Design review of the part built by this model. Coordinates are the model's own, in mm. A direction names the side the tool comes from. Round coordinates to 2 decimals unless told otherwise and drop trailing zeros. Order: outer loops, then holes, each group sorted by start corner. A loop starts at its lowest first (then second) coordinate and runs counter-clockwise, first axis right, second up.
from build123d import *

# Parameters (mm, degrees)
F0_R           = 11
F0_R_2         = 2.5
F1_DEPTH       = 7
F2_D           = 5.5
F2_CSINK_D     = 11.2
F2_CSINK_ANGLE = 90
F4_DEPTH       = 36
F5_SIZE        = 32


with BuildPart() as f1:
    # F0 (on Front) → F1 (new body)
    with BuildSketch(Plane.XZ):
        with BuildLine():
            Line((0, -33), (127, -33))
            Line((127, -33), (127, 33))
            Line((127, 33), (-33, 33))
            Line((-33, 33), (-33, 0))
            ThreePointArc((-33, 0), (-23.3345237792, -23.3345237792), (0, -33))
        make_face()
        Circle(F0_R, mode=Mode.SUBTRACT)
        with Locations((67, 10)):
            Circle(F0_R_2, mode=Mode.SUBTRACT)
        with Locations((92, 10)):
            Circle(F0_R_2, mode=Mode.SUBTRACT)
        with Locations((117, 10)):
            Circle(F0_R_2, mode=Mode.SUBTRACT)
    extrude(amount=-F1_DEPTH)

    # F2 (through all)
    with Locations(Plane.XZ):
        with Locations((117, 10), (92, 10), (67, 10)):
            CounterSinkHole(F2_D / 2, F2_CSINK_D / 2, counter_sink_angle=F2_CSINK_ANGLE)

    # F3 (on face) → F4 (join)
    with BuildSketch(Plane.XY.offset(33)):
        Polygon((0, 35), (-33, 35), (-33, 0), (127, 0), (127, 7), align=None)
    extrude(amount=F4_DEPTH)

    # F5
    f5_edges = [f1.edges().sort_by_distance(p)[0] for p in [
        (63.5, 21, 69),
    ]]
    chamfer(f5_edges, length=F5_SIZE)


solid = f1.part
1) Take a section at A-A on z = -7.5. Give the boundary of the cut face in (x, y), plus the area to 3 significant figures.
Results:
outline: (-32.14, 0) - (-8.05, 0) - (-8.05, 7) - (-32.14, 7) - close; (8.05, 0) - (127, 0) - (127, 7) - (8.05, 7) - close
area: 1,000 mm2
2) Take a section at D-D on x = 117. Give the boundary of the cut face in (y, z).
Results:
outline: (0, -33) - (7, -33) - (7, 7.25) - (2.85, 7.25) - (0, 4.4) - close; (0, 15.6) - (2.85, 12.75) - (7, 12.75) - (7, 33) - (9.2, 33) - (9.2, 37) - (0, 45.99) - close
3) Clearance check with flat-ended pins moving along their axes: P1, Ø5, axis at x = 117, z = 10, coming from the +Y side; P2, Ø6, axis at x = -1.5, y = 23.5, coming from the -Z side; P3, Ø7, axis at x = 67, z = 10, coming from the -Y side; P4, Ø1, axis at x = -9.5, y = 21.5, coming from the +Z side. State where each tip first meets the part, or that it passes through.
Results:
P1: passes through
P2: stops at z = 33
P3: stops at y = 2.1
P4: stops at z = 52.73
4) To check wall thickness, follow line 1 along X through (y, z) = (5.6, 10); line 2 along Y through (x, z) = (109, 10); line 3 along Z through (x, y) = (117, 3.9). State the ranges of each line that lie inside material, in increasing order.
Results:
line 1: x = -33 to -4.58, 4.58 to 64.25, 69.75 to 89.25, 94.75 to 114.25, 119.75 to 127
line 2: y = 0 to 7
line 3: z = -33 to 7.25, 12.75 to 42.18
5) Take a section at C-C on x = -22.5. Give the boundary of the cut face in (y, z), plus the area to 3 significant figures.
Results:
outline: (0, -24.14) - (7, -24.14) - (7, 33) - (35, 33) - (35, 41.84) - (7.19, 69) - (0, 69) - close
area: 1,280 mm2
6) The part is to be moulded in two halves that separate along X. For faces 3 (the face through (-33, 14, 42)), 4 (the face through (69.747, 4.954, 10.121)), 5 (the face through (63, 3, -33)), say which applies: released by +X, released by -X, zero draft, split by the parting line, or undercut.
Results:
face 3: released by -X
face 4: undercut
face 5: zero draft
7) For faces 1 (the face through (46, 7, 0)), 2 (the face through (119.747, 4.954, 10.121)), list the 3-axis set-ups (+Z, -Z, +X, -X, +Y, -Y) from which the entire face can be reached by the end or side of a thin tool; tool diameter is ignored.
Results:
face 1: -Z, +X, -X, +Y
face 2: +Y, -Y
8) Take a section at B-B on x = 92. Give the boundary of the cut face in (y, z), plus the area to 3 significant figures.
Results:
outline: (0, -33) - (7, -33) - (7, 7.25) - (2.85, 7.25) - (0, 4.4) - close; (0, 15.6) - (2.85, 12.75) - (7, 12.75) - (7, 33) - (14.72, 33) - (14.72, 37) - (0, 51.37) - close
area: 580 mm2
